The figure shows three views and two pictorial views of one solid part (mm, origin at its lowest corner). Answer the questions. A direction names the side the tool comes from. Round coordinates to 2 decimals unless told otherwise and drop trailing zeros. Order: outer loops, then holes, each group sorted by start corner. A loop starts at its lowest first (then second) coordinate and runs counter-clockwise, first axis right, second up. Notation, with made-up numbers: (-17, 65.5) -> (42, 65.5) arc R22 cw to (42, 94.5) -> close; hole circle Ø5 at (14, -38.5). An arc over 180 degrees is marked (long way). Answer as a JSON object with one key per item and string values. Group by question number.
Item 1: Section D-D, the plane y = 13 is taken. Write down the section's boundary in (x, z).
Item 2: Given P1, Ø1.9, axis at x = 7.5, z = 28.5, coming from the +Y side; P2, Ø2, axis at x = 17, y = 5, coming from the +Z side; P3, Ø5.5, axis at x = 12.5, z = 38.5, coming from the +Y side, each flat-ended and moving along its own axis, determine where each tip first touches the part or whether it passes through.
Item 3: Section A-A, the plane y = 3.75 is taken. Write down the section's boundary in (x, z), plus the area to 3 significant figures.
Item 4: Consider probe 1 along Z at (x, y) = (9.5, 13.75); probe 2 along X at (y, z) = (6.5, 12); probe 3 along X at (y, z) = (2.5, 21.5). Determine where each line is inside the solid, lowest interval first. Write a range as from..to.
Item 5: Section B-B, the plane x = 4.5 is taken. Write down the section's boundary in (y, z), plus the area to 4 significant figures.
Item 6: Section C-C, the plane z = 40 is taken. Write down the section's boundary in (x, y), plus the area to 3 significant figures.
Item 7: For the marked faces 1, 2 and 3, determine the directions among +Z, -Z, +X, -X, +Y, -Y from which every point of the face is accessible in a straight line to the end or side of a thin tool.
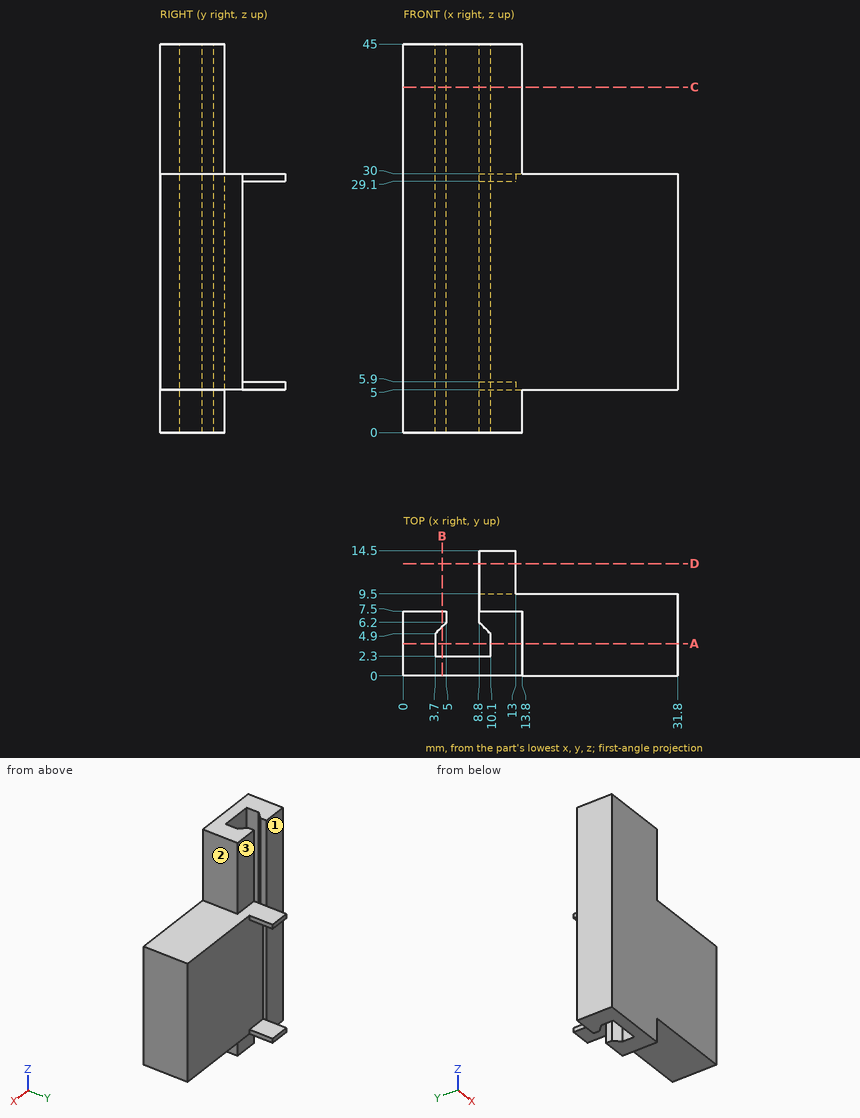
Values found:
{
 "1": {"outline": "(8.8, 5) -> (13, 5) -> (13, 5.9) -> (8.8, 5.9) -> close; (8.8, 29.1) -> (13, 29.1) -> (13, 30) -> (8.8, 30) -> close"},
 "2": {"P1": "y = 2.3", "P2": "z = 30", "P3": "y = 7.5"},
 "3": {"outline": "(0, 0) -> (3.7, 0) -> (3.7, 45) -> (0, 45) -> close; (10.1, 0) -> (13.8, 0) -> (13.8, 5) -> (31.8, 5) -> (31.8, 30) -> (13.8, 30) -> (13.8, 45) -> (10.1, 45) -> close", "area": "783 mm2"},
 "4": {"probe 1": "5..5.9, 29.1..30", "probe 2": "0..5, 8.8..31.8", "probe 3": "0..3.7, 10.1..31.8"},
 "5": {"outline": "(0, 0) -> (2.3, 0) -> (2.3, 45) -> (0, 45) -> close; (5.7, 0) -> (7.5, 0) -> (7.5, 45) -> (5.7, 45) -> close", "area": "184.5 mm2"},
 "6": {"outline": "(0, 0) -> (13.8, 0) -> (13.8, 7.5) -> (8.8, 7.5) -> (8.8, 6.2) -> (10.1, 4.9) -> (10.1, 2.3) -> (3.7, 2.3) -> (3.7, 4.9) -> (5, 6.2) -> (5, 7.5) -> (0, 7.5) -> close", "area": "75.3 mm2"},
 "7": {"face 1": "+Z, -Z, -X, +Y", "face 2": "+Z, +X, +Y, -Y", "face 3": "+Z, +X, -X, +Y"}
}
